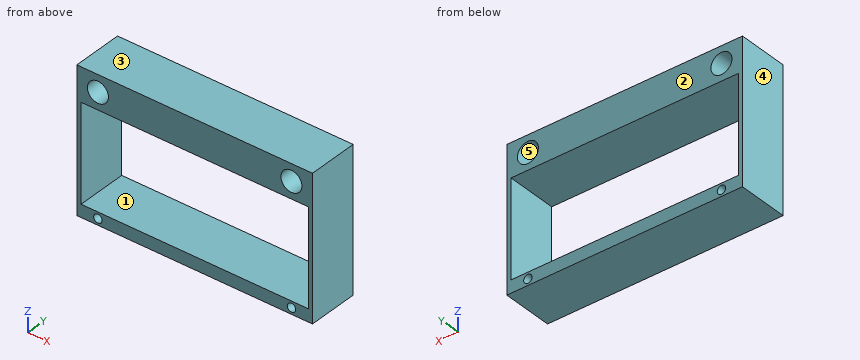
from build123d import *

# Parameters (mm, degrees)
EXTRUDE_1_DEPTH     = 12
SKETCH_4_W          = 56
SKETCH_4_H          = 2
EXTRUDE_2_DEPTH     = 12
SKETCH_3_R          = 2.5
SKETCH_3_R_2        = 1
CUT_EXTRUDE_1_DEPTH = 52.777268973


with BuildPart() as part:
    # 草图2 → 凸台-拉伸1 (new body)
    with BuildSketch(Plane(origin=(0, 0, 0), x_dir=(1, 0, 0), z_dir=(0, 1, 0))):
        Polygon((-10.725663717, 9.92920354), (45.274336283, 9.92920354), (45.274336283, -22.07079646), (-10.725663717, -22.07079646), (-10.725663717, -7.07079646), (-10.725663717, 1.92920354), align=None)
        Polygon((-9.725663717, -7.07079646), (-9.725663717, -14.07079646), (44.274336283, -14.07079646), (44.274336283, 8.92920354), (-9.725663717, 8.92920354), (-9.725663717, 0.92920354), align=None, mode=Mode.SUBTRACT)
    extrude(amount=EXTRUDE_1_DEPTH)

    # 草图4 → 凸台-拉伸2 (add)
    with BuildSketch(Plane(origin=(0, 0, 0), x_dir=(1, 0, 0), z_dir=(0, 1, 0))):
        with Locations((17.274336283, 10.92920354)):
            Rectangle(SKETCH_4_W, SKETCH_4_H)
    extrude(amount=EXTRUDE_2_DEPTH)

    # 草图3 → 切除-拉伸1 (cut, through all)
    with BuildSketch(Plane(origin=(0, 12, 0), x_dir=(1, 0, 0), z_dir=(0, 1, 0))):
        with Locations(Location((-5.725663717, -18.07079646, 0), (0, 0, 270))):
            Circle(SKETCH_3_R)
        with Locations(Location((40.274336283, -18.07079646, 0), (0, 0, 270))):
            Circle(SKETCH_3_R)
        with Locations(Location((-5.725663717, 10.42920354, 0), (0, 0, 270))):
            Circle(SKETCH_3_R_2)
        with Locations(Location((40.274336283, 10.42920354, 0), (0, 0, 270))):
            Circle(SKETCH_3_R_2)
    extrude(amount=-CUT_EXTRUDE_1_DEPTH, mode=Mode.SUBTRACT)


solid = part.part
Check sheet for the modelled part. Datum: model origin and axes. Units: mm. Face numbers are marked on the shaded views. A direction names the side the tool comes from. Round coordinates to 2 decimals unless told otherwise and drop trailing zeros. Loops run counter-clockwise (first coordinate to the right, second up) from the corner with the lowest first, then second, coordinate; pieces in that order, holes last. Notation, with made-up numbers: M 63.25,63.25 L 83.25,63.25 A7 cw 83.25,74.25 Z; hole C -37.75,-35 d9. An arc over 180 degrees is marked long. One line per item, written item: value.
(1) Sectioned sample at A-A, the plane x = 13. Record the cut outline in (y, z).
Computed values:
outline: M 0,-11.93 L 12,-11.93 L 12,-8.93 L 0,-8.93 Z; M 0,14.07 L 12,14.07 L 12,22.07 L 0,22.07 Z
(2) Release check for a two-part mould opening along X. For the marked faces 3, 4 and 5 record: +X half, -X half, draft (parallel to the pull), parting line (faces both ways), or undercut.
Computed values:
face 3: draft
face 4: -X half
face 5: undercut
(3) Sectioned sample at B-B, the plane z = 7.5. Record the cut outline in (x, y), then the cut area to 3 significant figures.
Computed values:
outline: M -10.73,0 L -9.73,0 L -9.73,12 L -10.73,12 Z; M 44.27,0 L 45.27,0 L 45.27,12 L 44.27,12 Z
area: 24.0 mm^2
(4) Sectioned sample at C-C, the plane y = 6. Record the cut outline in (x, z), then the cut area to 3 significant figures.
Computed values:
outline: M -10.73,-11.93 L 45.27,-11.93 L 45.27,22.07 L -10.73,22.07 Z; hole M -9.73,-8.93 L 44.27,-8.93 L 44.27,14.07 L -9.73,14.07 Z; hole C -5.73,18.07 d5; hole C -5.73,-10.43 d2; hole C 40.27,18.07 d5; hole C 40.27,-10.43 d2
area: 616 mm^2
(5) Access from +Z, -Z, +X, -X, +Y, -Y to the whole of each face (thin tool, end or side, straight path). Record for the marked faces 1 and 2.
Computed values:
face 1: +Y, -Y
face 2: +Z, -Z, +X, -X, +Y
(6) Depth check by flat-ended pin: pin 1 Ø4 at (x, z) = (40.27, 18.07) entering from +Y. Enter the tip coordinate at first touch or a pass-through.
Computed values:
pin 1: passes through
(7) Thickness scan on line 1 (X direction, y = 4.5, z = 18); line 2 (X direction, y = 7.75, z = -3); line 3 (Z direction, x = 31, y = 4.5). Record the ranges inside material, lowest first.
Computed values:
line 1: x = -10.73 to -8.22, -3.23 to 37.78, 42.77 to 45.27
line 2: x = -10.73 to -9.73, 44.27 to 45.27
line 3: z = -11.93 to -8.93, 14.07 to 22.07
